from build123d import *

# Parameters (mm, degrees)
BOSS_EXTRUDE1_DEPTH = 1
CUT_EXTRUDE2_DEPTH  = 1
SKETCH3_R           = 1.5
CUT_EXTRUDE3_DEPTH  = 1
BOSS_EXTRUDE2_START = -1
BOSS_EXTRUDE2_DEPTH = 1
BOSS_EXTRUDE3_DEPTH = 1
SKETCH6_R           = 1.5
SKETCH6_W           = 9
SKETCH6_H           = 30
SKETCH6_W_2         = 30
SKETCH6_H_2         = 9
CUT_EXTRUDE4_DEPTH  = 1
CUT_EXTRUDE5_DEPTH  = 1
SKETCH8_W           = 50
SKETCH8_H           = 20
CUT_EXTRUDE6_DEPTH  = 1


with BuildPart() as part:
    # Sketch1 → Boss-Extrude1 (new body)
    with BuildSketch(Plane(origin=(0, 0, 0), x_dir=(1, 0, 0), z_dir=(0, 1, 0))):
        with BuildLine():
            Line((1, 0), (99, 0))
            ThreePointArc((99, 0), (99.707106781, 0.292893219), (100, 1))
            Line((100, 1), (100, 99))
            ThreePointArc((100, 99), (99.707106781, 99.707106781), (99, 100))
            Line((99, 100), (1, 100))
            ThreePointArc((1, 100), (0.292893219, 99.707106781), (0, 99))
            Line((0, 99), (0, 1))
            ThreePointArc((0, 1), (0.292893219, 0.292893219), (1, 0))
        make_face()
        with BuildLine():
            Line((10, 21.5), (90, 21.5))
            ThreePointArc((90, 21.5), (91.5, 20), (90, 18.5))
            Line((90, 18.5), (10, 18.5))
            ThreePointArc((10, 18.5), (8.5, 20), (10, 21.5))
        make_face(mode=Mode.SUBTRACT)
    extrude(amount=BOSS_EXTRUDE1_DEPTH)

    # Sketch2 → Cut-Extrude2 (cut)
    with BuildSketch(Plane(origin=(0, 1, 0), x_dir=(1, 0, 0), z_dir=(0, 1, 0))):
        with BuildLine():
            Line((0, 100), (0, 65))
            Line((0, 65), (19, 65))
            ThreePointArc((19, 65), (19.707106781, 65.292893219), (20, 66))
            Line((20, 66), (20, 100))
            Line((20, 100), (0, 100))
        make_face()
        with BuildLine():
            Line((100, 65), (100, 100))
            Line((100, 100), (80, 100))
            Line((80, 100), (80, 66))
            ThreePointArc((80, 66), (80.292893219, 65.292893219), (81, 65))
            Line((81, 65), (100, 65))
        make_face()
    extrude(amount=-CUT_EXTRUDE2_DEPTH, mode=Mode.SUBTRACT)

    # Sketch3 → Cut-Extrude3 (cut)
    with BuildSketch(Plane(origin=(0, 1, 0), x_dir=(1, 0, 0), z_dir=(0, 1, 0))):
        with Locations(Location((6, 26, 0), (0, 0, 270))):
            Circle(SKETCH3_R)
        with Locations(Location((23, 95, 0), (0, 0, 270))):
            Circle(SKETCH3_R)
        with Locations(Location((77, 95, 0), (0, 0, 270))):
            Circle(SKETCH3_R)
        with Locations(Location((94, 26, 0), (0, 0, 270))):
            Circle(SKETCH3_R)
        with Locations(Location((6, 62, 0), (0, 0, 270))):
            Circle(SKETCH3_R)
        with Locations(Location((94, 62, 0), (0, 0, 270))):
            Circle(SKETCH3_R)
    extrude(amount=-CUT_EXTRUDE3_DEPTH, mode=Mode.SUBTRACT)

    # Sketch4 → Boss-Extrude2 (add)
    with BuildSketch(Plane(origin=(0, 1, 0), x_dir=(1, 0, 0), z_dir=(0, 1, 0)).offset(BOSS_EXTRUDE2_START)):
        with BuildLine():
            Line((0, 1), (0, -10))
            Line((0, -10), (100, -10))
            Line((100, -10), (100, 1))
            ThreePointArc((100, 1), (99.707106781, 0.292893219), (99, 0))
            Line((99, 0), (1, 0))
            ThreePointArc((1, 0), (0.292893219, 0.292893219), (0, 1))
        make_face()
    extrude(amount=BOSS_EXTRUDE2_DEPTH)

    # Sketch5 → Boss-Extrude3 (add)
    with BuildSketch(Plane(origin=(0, 1, 0), x_dir=(1, 0, 0), z_dir=(0, 1, 0))):
        with BuildLine():
            Line((100, 65), (128, 65))
            ThreePointArc((128, 65), (129.414213562, 64.414213562), (130, 63))
            Line((130, 63), (130, 26.5))
            ThreePointArc((130, 26.5), (129.414213562, 25.085786438), (128, 24.5))
            Line((128, 24.5), (100, 24.5))
            Line((100, 24.5), (100, 65))
        make_face()
        with BuildLine():
            Line((0, 24.5), (-28, 24.5))
            ThreePointArc((-28, 24.5), (-29.414213562, 25.085786438), (-30, 26.5))
            Line((-30, 26.5), (-30, 63))
            ThreePointArc((-30, 63), (-29.414213562, 64.414213562), (-28, 65))
            Line((-28, 65), (0, 65))
            Line((0, 65), (0, 24.5))
        make_face()
        with BuildLine():
            Line((80, 100), (20, 100))
            Line((20, 100), (20, 128))
            ThreePointArc((20, 128), (20.585786438, 129.414213562), (22, 130))
            Line((22, 130), (78, 130))
            ThreePointArc((78, 130), (79.414213562, 129.414213562), (80, 128))
            Line((80, 128), (80, 100))
        make_face()
    extrude(amount=-BOSS_EXTRUDE3_DEPTH)

    # Sketch6 → Cut-Extrude4 (cut)
    with BuildSketch(Plane(origin=(0, 1, 0), x_dir=(1, 0, 0), z_dir=(0, 1, 0))):
        with Locations(Location((31.5, 3.5, 0), (0, 0, 270))):
            Circle(SKETCH6_R)
        with Locations(Location((-15, 62.75, 0), (0, 0, 270))):
            Circle(SKETCH6_R)
        with Locations(Location((-15, 26.75, 0), (0, 0, 90))):
            Circle(SKETCH6_R)
        with Locations(Location((68.5, 3.5, 0), (0, 0, 90))):
            Circle(SKETCH6_R)
        with Locations(Location((115, 26.75, 0), (0, 0, 270))):
            Circle(SKETCH6_R)
        with Locations(Location((115, 62.75, 0), (0, 0, 90))):
            Circle(SKETCH6_R)
        with Locations((115, 44.75)):
            Rectangle(SKETCH6_W, SKETCH6_H)
        with Locations((-15, 44.75)):
            Rectangle(SKETCH6_W, SKETCH6_H)
        with Locations((50, 3.5)):
            Rectangle(SKETCH6_W_2, SKETCH6_H_2)
    extrude(amount=-CUT_EXTRUDE4_DEPTH, mode=Mode.SUBTRACT)

    # Sketch7 → Cut-Extrude5 (cut)
    with BuildSketch(Plane(origin=(0, 1, 0), x_dir=(1, 0, 0), z_dir=(0, 1, 0))):
        with BuildLine():
            Line((0, 24.5), (2.972707359, 24.5))
            ThreePointArc((2.972707359, 24.5), (3.972707359, 23.5), (2.972707359, 22.5))
            Line((2.972707359, 22.5), (0, 22.5))
            ThreePointArc((0, 22.5), (-1, 23.5), (0, 24.5))
        make_face()
        with BuildLine():
            Line((19.996436831, 101), (23.359178087, 101))
            ThreePointArc((23.359178087, 101), (24.859178087, 99.5), (23.359178087, 98))
            Line((23.359178087, 98), (19.996436831, 98))
            ThreePointArc((19.996436831, 98), (18.496436831, 99.5), (19.996436831, 101))
        make_face()
        with BuildLine():
            Line((1.2, 24.5), (1.2, 27.556784127))
            ThreePointArc((1.2, 27.556784127), (2.2, 28.556784127), (3.2, 27.556784127))
            Line((3.2, 27.556784127), (3.2, 24.5))
            ThreePointArc((3.2, 24.5), (2.2, 23.5), (1.2, 24.5))
        make_face()
        with BuildLine():
            Line((1.2, 65), (1.2, 61.943215873))
            ThreePointArc((1.2, 61.943215873), (2.2, 60.943215873), (3.2, 61.943215873))
            Line((3.2, 61.943215873), (3.2, 65))
            ThreePointArc((3.2, 65), (2.2, 66), (1.2, 65))
        make_face()
        with BuildLine():
            Line((80.003563169, 101), (76.640821913, 101))
            ThreePointArc((76.640821913, 101), (75.140821913, 99.5), (76.640821913, 98))
            Line((76.640821913, 98), (80.003563169, 98))
            ThreePointArc((80.003563169, 98), (81.503563169, 99.5), (80.003563169, 101))
        make_face()
        with BuildLine():
            Line((98.8, 24.5), (98.8, 27.556784127))
            ThreePointArc((98.8, 27.556784127), (97.8, 28.556784127), (96.8, 27.556784127))
            Line((96.8, 27.556784127), (96.8, 24.5))
            ThreePointArc((96.8, 24.5), (97.8, 23.5), (98.8, 24.5))
        make_face()
        with BuildLine():
            Line((100, 24.5), (97.027292641, 24.5))
            ThreePointArc((97.027292641, 24.5), (96.027292641, 23.5), (97.027292641, 22.5))
            Line((97.027292641, 22.5), (100, 22.5))
            ThreePointArc((100, 22.5), (101, 23.5), (100, 24.5))
        make_face()
        with BuildLine():
            Line((98.8, 65), (98.8, 61.943215873))
            ThreePointArc((98.8, 61.943215873), (97.8, 60.943215873), (96.8, 61.943215873))
            Line((96.8, 61.943215873), (96.8, 65))
            ThreePointArc((96.8, 65), (97.8, 66), (98.8, 65))
        make_face()
    extrude(amount=-CUT_EXTRUDE5_DEPTH, mode=Mode.SUBTRACT)

    # Sketch8 → Cut-Extrude6 (cut)
    with BuildSketch(Plane(origin=(0, 1, 0), x_dir=(1, 0, 0), z_dir=(0, 1, 0))):
        with Locations((50, 44)):
            Rectangle(SKETCH8_W, SKETCH8_H)
    extrude(amount=-CUT_EXTRUDE6_DEPTH, mode=Mode.SUBTRACT)


solid = part.part
The listing builds one solid part. Answer for the finished solid, in the listing's coordinates (mm). Coordinates: 2 decimals unless noted, no trailing zeros. Loops run counter-clockwise (first coordinate to the right, second up) from the corner with the lowest first, then second, coordinate; pieces in that order, holes last. Notation, with made-up numbers: (44, 25) -> (64, 25) arc R27 ccw to (64, 59) -> close; hole circle Ø11 at (59, -21). An arc over 180 degrees is marked (long way). Write item = value, one per line. Start each with the question number.
1) A cutting plane is placed at C-C (z = -103). Give the vertices of the cut face in (x, y).
2) Straight lines are drawn through the part: line 1 (Z direction, x = 27, y = 0.7); line 2 (Z direction, x = 68.5, y = 0.4); line 3 (X direction, y = 0.3, z = -95). For each, find the intervals that lie inside material, in ascending order. Write a range as from..to.
3) A cutting plane is placed at A-A (z = -46). Give the vertices of the cut face in (x, y).
4) A cutting plane is placed at B-B (y = 0.45). Count the separate pieces of the cut face and the enclosed holes in it, then the cut area to 3 significant figures.
5) Given pin 1 Ø2.5 at (x, z) = (68.5, -3.5) entering from +Y; pin 2 Ø0.5 at (x, y) = (114.5, 0.5) entering from +Z, each flat-ended and moving along its own axis, determine where each tip first touches the part or whether it passes through.
Responses:
q1.outline = (20, 0) -> (80, 0) -> (80, 1) -> (20, 1) -> close
q2.line_1 = -130..-54, -34..-21.5, -18.5..10
q2.line_2 = -130..-54, -34..-21.5, -18.5..-5, -2..10
q2.line_3 = 20..21.5, 24.5..75.5, 78.5..80
q3.outline = (-30, 0) -> (-19.5, 0) -> (-19.5, 1) -> (-30, 1) -> close; (-10.5, 0) -> (25, 0) -> (25, 1) -> (-10.5, 1) -> close; (75, 0) -> (110.5, 0) -> (110.5, 1) -> (75, 1) -> close; (119.5, 0) -> (130, 0) -> (130, 1) -> (119.5, 1) -> close
q4.separate_pieces = 1
q4.enclosed_holes = 17
q4.area = 11,600 mm²
q5.pin_1 = through
q5.pin_2 = -24.5
